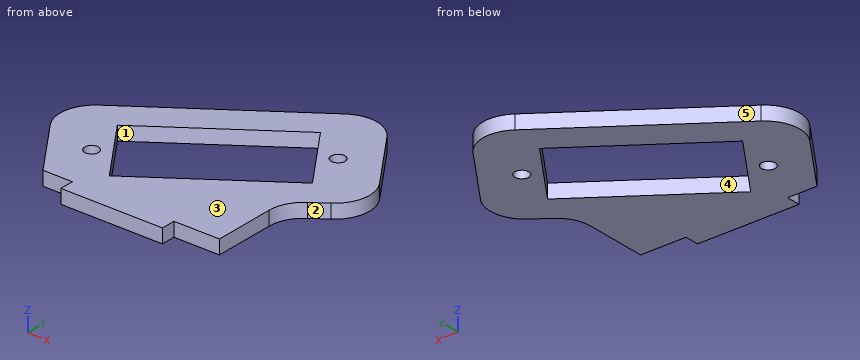
```python
from build123d import *

# Parameters (mm, degrees)
SKETCH1_R           = 1
BOSS_EXTRUDE1_DEPTH = 2


with BuildPart() as part:
    # Sketch1 → Boss-Extrude1 (new body)
    with BuildSketch(Plane.XY):
        with BuildLine():
            Line((0, 0), (14.5, 0))
            Line((14.5, 0), (14.5, 2))
            Line((14.5, 2), (21, 2))
            Line((21, 2), (21, 10.652873099))
            ThreePointArc((21, 10.652873099), (21.564945834, 12.961616165), (23.132117818, 14.74863332))
            Line((23.132117818, 14.74863332), (25.264156906, 16.241503161))
            ThreePointArc((25.264156906, 16.241503161), (27.320313489, 19.469022494), (26.492034945, 23.205145564))
            Line((26.492034945, 23.205145564), (20.297409433, 32.051987643))
            ThreePointArc((20.297409433, 32.051987643), (17.0698901, 34.108144226), (13.33376703, 33.279865682))
            Line((13.33376703, 33.279865682), (-9.02908378, 17.62122897))
            ThreePointArc((-9.02908378, 17.62122897), (-11.085240363, 14.393709637), (-10.256961819, 10.657586567))
            Line((-10.256961819, 10.657586567), (-4.194854443, 2))
            Line((-4.194854443, 2), (0, 2))
            Line((0, 2), (0, 0))
        make_face()
        with Locations((-3.063888841, 9.102047709)):
            Circle(SKETCH1_R, mode=Mode.SUBTRACT)
        with Locations((19.298961968, 24.760684422)):
            Circle(SKETCH1_R, mode=Mode.SUBTRACT)
        Polygon((-4.48202491, 15.311628218), (13.948896087, 28.217098036), (20.717098036, 18.551103913), (2.286177039, 5.645634095), align=None, mode=Mode.SUBTRACT)
    extrude(amount=BOSS_EXTRUDE1_DEPTH)


solid = part.part
```
Input: part model. Units: mm. Frame: model coordinates. Face numbers are marked on the shaded views. A direction names the side the tool comes from. Give positions to 0.01 mm unless a question says otherwise; leave off trailing zeros. Order: outer loops, then holes, each group sorted by start corner. A loop starts at its lowest first (then second) coordinate and runs counter-clockwise, first axis right, second up. Notation, with made-up numbers: (78, 70.5) - (134, 70.5) arc R26 cw to (134, 89.5) - close; hole circle Ø2 at (14.5, 83). An arc over 180 degrees is marked (long way). Use a Markdown table: item, result.
(1) Section query C-C (z = 1.1). Output: boundary loops of the cut face in (x, y).
Computed values:
| item | result |
|---|---|
| outline | (-10.26, 10.66) - (-4.19, 2) - (0, 2) - (0, 0) - (14.5, 0) - (14.5, 2) - (21, 2) - (21, 10.65) arc R5 cw to (23.13, 14.75) - (25.26, 16.24) arc R5 ccw to (26.49, 23.21) - (20.3, 32.05) arc R5 ccw to (13.33, 33.28) - (-9.03, 17.62) arc R5 ccw to start; hole (-4.48, 15.31) - (2.29, 5.65) - (20.72, 18.55) - (13.95, 28.22) - close; hole circle Ø2 at (-3.06, 9.1); hole circle Ø2 at (19.3, 24.76) |
(2) Pin query (flat end, axial travel): pin 1 (0.6 mm diameter, centred on x = -2, z = 1, fed in from -Y); pin 2 (1 mm diameter, centred on y = 1, z = 1, fed in from +X); pin 3 (1 mm diameter, centred on y = 7, z = 0.5, fed in from +X). Return the tip coordinate at first contact, or that it passes through.
Computed values:
| item | result |
|---|---|
| pin 1 | stops at y = 2 |
| pin 2 | stops at x = 14.5 |
| pin 3 | stops at x = 21 |
(3) Section query B-B (y = 20). Output: boundary loops of the cut face in (x, z), then the cut area to 3 significant figures.
Computed values:
| item | result |
|---|---|
| outline | (-5.63, 0) - (2.21, 0) - (2.21, 2) - (-5.63, 2) - close; (19.7, 0) - (27.38, 0) - (27.38, 2) - (19.7, 2) - close |
| area | 31.1 mm2 |
(4) Draft query along X for the marked faces 1, 2 and 3. Return one class per face: released by +X, released by -X, zero draft, split by the parting line, or undercut.
Computed values:
| item | result |
|---|---|
| face 1 | undercut |
| face 2 | released by +X |
| face 3 | zero draft |
(5) Section query A-A (x = 4). Output: boundary loops of the cut face in (y, z), then the cut area to 3 significant figures.
Computed values:
| item | result |
|---|---|
| outline | (0, 0) - (6.85, 0) - (6.85, 2) - (0, 2) - close; (21.25, 0) - (26.74, 0) - (26.74, 2) - (21.25, 2) - close |
| area | 24.7 mm2 |
(6) Line query: line 1 (Y direction, x = 18.5, z = 0.4); line 2 (X direction, y = 24.5, z = 1.8); line 3 (Y direction, x = 11, z = 0.85). Output: solid intervals per line, ascending. Write a range as from..to.
Computed values:
| item | result |
|---|---|
| line 1 | y = 2..17, 21.72..24.16, 25.36..33.62 |
| line 2 | x = 0.79..8.64, 16.55..18.33, 20.26..25.59 |
| line 3 | y = 0..11.75, 26.15..31.65 |
(7) Access query for the marked faces 4 and 5. Directions: +Z, -Z, +X, -X, +Y, -Y. A direction counts if a zero-diameter tool reaches every point of the face in a straight line with its end or side. Return the directions, or none.
Computed values:
| item | result |
|---|---|
| face 4 | +Z, -Z |
| face 5 | +Z, -Z, -X, +Y |
(8) Section query D-D (y = 31.5). Output: boundary loops of the cut face in (x, z).
Computed values:
| item | result |
|---|---|
| outline | (10.79, 0) - (20.68, 0) - (20.68, 2) - (10.79, 2) - close |
